Here's how the part is built. I have some questions about the finished solid (model axes, mm). Give positions to 0.01 mm unless a question says otherwise; leave off trailing zeros. Order: outer loops, then holes, each group sorted by start corner. A loop starts at its lowest first (then second) coordinate and runs counter-clockwise, first axis right, second up. Notation, with made-up numbers: M 12,80.5 L 25,80.5 A15 ccw 25,95.5 Z; hole C 38.25,3.5 d4. An arc over 180 degrees is marked long. One line per item, written item: value. Start each with the question number.
from build123d import *

# Parameters (mm, degrees)
BLANKSKE_W         = 165
BLANKSKE_H         = 9.5
BLANK_DEPTH        = 13
TOOTHCUTSIM_DEPTH  = 166.78374468
TEETHCUTS_COUNT    = 27
TEETHCUTS_PITCH    = 6.2831853
ESQUISSE1_W        = 165
ESQUISSE1_H        = 20
BOSS_EXTRU_1_DEPTH = 7


with BuildPart() as part:
    # BlankSke → Blank (new body)
    with BuildSketch(Plane.XY):
        with Locations((82.5, 4.75)):
            Rectangle(BLANKSKE_W, BLANKSKE_H)
    extrude(amount=-BLANK_DEPTH)

    # TooCutSkeSim → ToothCutSim (cut, through all)
    with BuildSketch(Plane.XY):
        Polygon((0.861870739, 5), (-0.861870739, 5), (-2.508981637, 9.5254), (2.508981637, 9.5254), align=None)
    toothcutsim = extrude(amount=-TOOTHCUTSIM_DEPTH, mode=Mode.SUBTRACT)

    # TeethCuts: ToothCutSim ×27
    with Locations(*[(i * TEETHCUTS_PITCH, 0, 0) for i in range(1, TEETHCUTS_COUNT)]):
        add(toothcutsim, mode=Mode.SUBTRACT)

    # Esquisse1 → Boss.-Extru.1 (add)
    with BuildSketch(Plane.XY):
        with Locations((82.5, 10)):
            Rectangle(ESQUISSE1_W, ESQUISSE1_H)
    extrude(amount=BOSS_EXTRU_1_DEPTH)


solid = part.part
Item 1: I want a section at A-A on y = 13. Write out the boundary of the cut face in (x, z).
Item 2: We'd pull the mould along X, two halves only. Please class faces 1 (the face through (70.807, 7.282, -6.409)), 2 (the face through (81, 0, -3)): +X half, -X half, draft (parallel to the pull), parting line (faces both ways), or undercut.
Item 3: Will these pins go through, and if not, where does the flat tip stop? P1, Ø1, axis at x = 53.5, z = -8, coming from the +Y side; P2, Ø1.4, axis at x = 100.5, z = -9, coming from the +Y side.
Item 4: Please list where these lines run through material, in increasing order: probe 1 along Z at (x, y) = (47.5, 12); probe 2 along Y at (x, z) = (100, -7.5). Write a range as [from, to].
Answer below:
1. outline: M 0,0 L 165,0 L 165,7 L 0,7 Z
2. face 1: undercut
2. face 2: draft
3. P1: stops at y = 9.5
3. P2: stops at y = 5
4. probe 1: z = [0, 7]
4. probe 2: y = [0, 5]
